Can you work these out from the model? Positions are in its coordinate system, mm. A direction names the side the tool comes from. Give positions to 0.01 mm unless a question says otherwise; leave off trailing zeros. Order: outer loops, then holes, each group sorted by start corner. A loop starts at its lowest first (then second) coordinate and runs counter-clockwise, first axis right, second up. Notation, with made-up numbers: M 55,10.25 L 89,10.25 A28 ccw 89,36.25 Z; hole C 87.25,81.25 d6. An arc over 180 degrees is marked long. Use one line per item in the form item = value. Start each with the question number.
1. I want a section at C-C, the plane y = 0. List the corners of the cut face in (x, z) for me, and give its area (3 significant figures).
2. I want a section at A-A, the plane y = 10. List the corners of the cut face in (x, z) for me.
3. I need wall thicknesses on L1, parallel to X at y = 0, z = -0.7; L2, parallel to Z at x = 1.7, y = 10; L3, parallel to Y at x = 15, z = -1.2. Which ranges of each line are inside material? Lowest first, please.
4. We'd pull the mould along Y, two halves only. Please class faces 4 (the face through (21.987, -14.248, -1.479)), 5 (the face through (1, 15, 1)), 6 (the face through (1.48, 8.38, 11.49)): +Y half, -Y half, draft (parallel to the pull), parting line (faces both ways), or undercut.
5. Will these pins go through, and if not, where does the flat tip stop? P1, Ø11, axis at x = -12, y = -6, coming from the +Z side; P2, Ø9, axis at y = -2, z = 14, coming from the +X side; P3, Ø5, axis at y = -4, z = 17.5, coming from the -X side; P4, Ø4, axis at y = -10, z = 10, coming from the -X side.
6. I want a section at D-D, the plane z = -0.5. List the corners of the cut face in (x, y) for me.
7. For faces 1 (the face through (14, -4, 0)), 2 (the face through (0, 0, 11)), 3 (the face through (21.987, 14.248, -1.479)), which set-ups out of +Z, -Z, +X, -X, +Y, -Y let a thin tool reach every point of the face, with its end or its side?
8. I want a section at B-B, the plane x = -15. List the corners of the cut face in (y, z) for me, and give its area (3 significant figures).
```python
from build123d import *

# Parameters (mm, degrees)
PAD_DEPTH            = 3
PAD_MIRRORED_2_DEPTH = 3
SKETCH001_R          = 2.2
PAD001_DEPTH         = 3
FILLET_R             = 1
FILLET001_R          = 3


with BuildPart() as part:
    # Sketch → Pad (new body)
    with BuildSketch(Plane.XY):
        with BuildLine():
            Line((0, 0), (12.3, 0))
            ThreePointArc((17.7, 0), (15, 2.7), (12.3, 0))
            Line((17.7, 0), (22.7, 0))
            Line((22.7, 0), (22.7, 12.5))
            ThreePointArc((22.7, 12.5), (21.967767, 14.267767), (20.2, 15))
            Line((20.2, 15), (0, 15))
            Line((0, 15), (0, 0))
        make_face()
    pad = extrude(amount=-PAD_DEPTH)

    # Sketch Mirrored 2 → Pad Mirrored 2 (add)
    with BuildSketch(Plane(origin=(0, 0, 0), x_dir=(-1, 0, 0), z_dir=(0, 0, -1))):
        with BuildLine():
            Line((0, 0), (12.3, 0))
            ThreePointArc((17.7, 0), (15, 2.7), (12.3, 0))
            Line((17.7, 0), (22.7, 0))
            Line((22.7, 0), (22.7, 12.5))
            ThreePointArc((22.7, 12.5), (21.967767, 14.267767), (20.2, 15))
            Line((20.2, 15), (0, 15))
            Line((0, 15), (0, 0))
        make_face()
    pad_mirrored_2 = extrude(amount=PAD_MIRRORED_2_DEPTH)

    # Mirrored001: Pad, Pad Mirrored 2 across Sketch H_Axis
    add(pad.mirror(Plane.ZX))
    add(pad_mirrored_2.mirror(Plane.ZX))

    # Sketch001 → Pad001 (join)
    with BuildSketch(Plane.YZ):
        with BuildLine():
            Line((0, 0), (15, 0))
            Line((15, 0), (15, 18.5))
            ThreePointArc((15, 18.5), (14.267767, 20.267767), (12.5, 21))
            Line((12.5, 21), (0, 21))
            Line((0, 21), (0, 0))
        make_face()
        with Locations((10, 10)):
            Circle(SKETCH001_R, mode=Mode.SUBTRACT)
    pad001 = extrude(amount=PAD001_DEPTH)

    # Mirrored002: Pad001 across Sketch001 V_Axis
    add(pad001.mirror(Plane(origin=(0, 0, 0), x_dir=(1, 0, 0), z_dir=(0, 1, 0))))

    # Fillet
    fillet_edges = [part.edges().sort_by_distance(p)[0] for p in [
        (0, -7.5, 0),
    ]]
    fillet(fillet_edges, radius=FILLET_R)

    # Fillet001
    fillet001_edges = [part.edges().sort_by_distance(p)[0] for p in [
        (3, -7.5, 0),
    ]]
    fillet(fillet001_edges, radius=FILLET001_R)


solid = part.part
```
Check result:
q1.outline = M -22.7,-3 L -17.7,-3 L -17.7,0 L -22.7,0 Z; M -12.3,-3 L 12.3,-3 L 12.3,0 L 6,0 A3 cw 3,3 L 3,21 L 0,21 L 0,1 A1 cw -1,0 L -12.3,0 Z; M 17.7,-3 L 22.7,-3 L 22.7,0 L 17.7,0 Z
q1.area = 169 mm2
q2.outline = M -22.7,-3 L 22.7,-3 L 22.7,0 L 6,0 A3 cw 3,3 L 3,7.8 L 0,7.8 L 0,1 A1 cw -1,0 L -22.7,0 Z; M 0,12.2 L 3,12.2 L 3,21 L 0,21 Z
q3.L1 = -22.7 to -17.7, -12.3 to 12.3, 17.7 to 22.7
q3.L2 = -3 to 7.8, 12.2 to 21
q3.L3 = -15 to -2.7, 2.7 to 15
q4.face_4 = -Y half
q4.face_5 = +Y half
q4.face_6 = undercut
q5.P1 = 0
q5.P2 = 3
q5.P3 = 0
q5.P4 = through
q6.outline = M -22.7,-12.5 A2.5 ccw -20.2,-15 L 20.2,-15 A2.5 ccw 22.7,-12.5 L 22.7,12.5 A2.5 ccw 20.2,15 L -20.2,15 A2.5 ccw -22.7,12.5 Z; hole C -15,0 d5.4; hole C 15,0 d5.4
q7.face_1 = +Z, +X, +Y, -Y
q7.face_2 = +Z, -X, +Y, -Y
q7.face_3 = +Z, -Z, +X, +Y
q8.outline = M -15,-3 L -2.7,-3 L -2.7,0 L -15,0 Z; M 2.7,-3 L 15,-3 L 15,0 L 2.7,0 Z
q8.area = 73.8 mm2
